Design review of the part shown in the three views and the two pictorial views. Dimensions are in mm from the part's minimum x, y and z. Coordinates: 2 decimals unless noted, no trailing zeros. Write each loop counter-clockwise with the first axis right and the second up, starting at its lowest first coordinate (ties: lowest second). Pieces come first, ordered by that corner, then holes. Notation, with made-up numbers: (46, 43) - (81, 43) arc R25 ccw to (81, 78) - close; hole circle Ø6 at (12.5, -5.5). An arc over 180 degrees is marked (long way). Answer as CSV lines item,"result". Start each with the question number.
Q1. For line 1 along Z through (x, y) = (12.7, 4); line 2 along X through (y, z) = (3.25, 88.9), list the stretches that pass through material, from the lowest coordinate up. Write a range as [from, to].
Q2. We need section B-B (z = 12.7). Write out the cut boundary in (x, y).
Q3. Clearance check with a flat-ended pin moving along its axis: pin 1 (4 mm diameter, centred on x = 88.9, z = 12.7, fed in from -Y). State where the tip first meets the part, or that it passes through.
Q4. We need section A-A (x = 12.7). Write out the cut boundary in (y, z), plus the area to 3 significant figures.
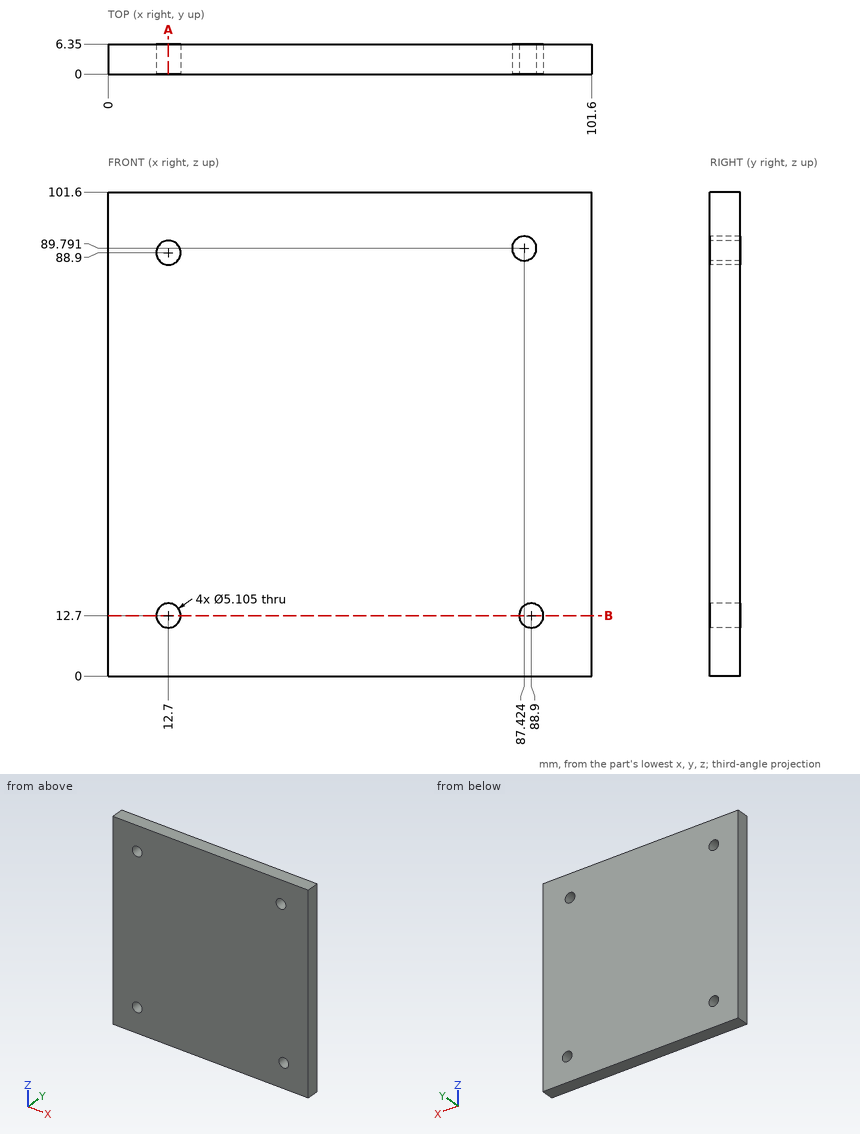
Results list:
1,line 1,"z = [0, 10.15], [15.25, 86.35], [91.45, 101.6]"
1,line 2,"x = [0, 10.15], [15.25, 85.03], [89.82, 101.6]"
2,outline,"(0, 0) - (10.15, 0) - (10.15, 6.35) - (0, 6.35) - close; (15.25, 0) - (86.35, 0) - (86.35, 6.35) - (15.25, 6.35) - close; (91.45, 0) - (101.6, 0) - (101.6, 6.35) - (91.45, 6.35) - close"
3,pin 1,"passes through"
4,outline,"(0, 0) - (6.35, 0) - (6.35, 10.15) - (0, 10.15) - close; (0, 15.25) - (6.35, 15.25) - (6.35, 86.35) - (0, 86.35) - close; (0, 91.45) - (6.35, 91.45) - (6.35, 101.6) - (0, 101.6) - close"
4,area,"580 mm2"
